For this review, take the finished solid that the model builds, in its own axes (mm). Coordinates: 2 decimals unless noted, no trailing zeros. Order: outer loops, then holes, each group sorted by start corner. A loop starts at its lowest first (then second) coordinate and runs counter-clockwise, first axis right, second up. Notation, with made-up numbers: (-7, -12.75) -> (34, -12.75) arc R17 ccw to (34, 17.25) -> close; hole circle Ø3 at (-18.5, -20.5). An arc over 180 degrees is marked (long way). Return JSON: item names as keys, results as strings. Group by question number.
Item 1: Take a section at A-A (z = -45). Write out the cut boundary in (x, y), then the cut area to 3 significant figures.
Item 2: Draft analysis for pull direction Z (two halves, no side actions). For faces 1 (the cylindrical face through (102.027, -0.986, -68.641)), 2 (the flat face through (-2, 0, 1)), 3 (the cylindrical face through (0.358, -0.986, -67.773)), state which applies: +Z half, -Z half, draft (parallel to the pull), parting line (faces both ways), or undercut.
Item 3: For line 1 along Z through (x, y) = (100, -1.35); line 2 along X through (y, z) = (-0.5, -46.5), list the stretches that pass through material, from the lowest coordinate up.
Item 4: Take a section at D-D (x = -100). Write out the cut boundary in (y, z), then the cut area to 3 significant figures.
Item 5: Take a section at B-B (x = 100). Write out the cut boundary in (y, z), then the cut area to 3 significant figures.
Item 6: Take a section at C-C (z = -70.5). Write out the cut boundary in (x, y).
```python
from build123d import *

# Parameters (mm, degrees)
F0_W     = 254
F0_H     = 150
F1_DEPTH = 2
F2_R     = 6.25
F3_DEPTH = 25
F5_D     = 5.5
F5_DEPTH = 13
F5_TIP   = 1.6523667023


with BuildPart() as f1:
    # F0 (on Front) → F1 (new body)
    with BuildSketch(Plane.XZ):
        Rectangle(F0_W, F0_H)
    extrude(amount=F1_DEPTH)

    # F2 (on face) → F3 (cut)
    with BuildSketch(Plane.XZ.offset(2)):
        with Locations((-97, -45)):
            Circle(F2_R)
    extrude(amount=-F3_DEPTH, mode=Mode.SUBTRACT)

    # F5
    with Locations(Plane.XZ.offset(2)):
        with Locations((-100, -70.5), (0, -70.5), (100, -70.5)):
            Hole(F5_D / 2, depth=F5_DEPTH)
            with Locations((0, 0, -(F5_DEPTH + F5_TIP / 2))):  # 118° drill point
                Cone(0, F5_D / 2, F5_TIP, mode=Mode.SUBTRACT)


solid = f1.part
```
Findings below:
{
 "1": {"outline": "(-127, -2) -> (-103.25, -2) -> (-103.25, 0) -> (-127, 0) -> close; (-90.75, -2) -> (127, -2) -> (127, 0) -> (-90.75, 0) -> close", "area": "483 mm2"},
 "2": {"face 1": "undercut", "face 2": "draft", "face 3": "undercut"},
 "3": {"line 1": "z = -75 to -73.25, -67.75 to 75", "line 2": "x = -127 to -103.07, -90.93 to 127"},
 "4": {"outline": "(-2, -75) -> (0, -75) -> (0, -73.25) -> (-2, -73.25) -> close; (-2, -67.75) -> (0, -67.75) -> (0, -50.48) -> (-2, -50.48) -> close; (-2, -39.52) -> (0, -39.52) -> (0, 75) -> (-2, 75) -> close", "area": "267 mm2"},
 "5": {"outline": "(-2, -75) -> (0, -75) -> (0, -73.25) -> (-2, -73.25) -> close; (-2, -67.75) -> (0, -67.75) -> (0, 75) -> (-2, 75) -> close", "area": "289 mm2"},
 "6": {"outline": "(-127, -2) -> (-102.75, -2) -> (-102.75, 0) -> (-127, 0) -> close; (-97.25, -2) -> (-2.75, -2) -> (-2.75, 0) -> (-97.25, 0) -> close; (2.75, -2) -> (97.25, -2) -> (97.25, 0) -> (2.75, 0) -> close; (102.75, -2) -> (127, -2) -> (127, 0) -> (102.75, 0) -> close"}
}
